```python
from build123d import *

# Parameters (mm, degrees)
SKETCH1_R           = 2
SKETCH1_R_2         = 2.5
SKETCH1_R_3         = 5.5
SKETCH1_R_4         = 1.75
SKETCH1_R_5         = 8.75
SKETCH1_R_6         = 16
BOSS_EXTRUDE1_DEPTH = 3


with BuildPart() as part:
    # Sketch1 → Boss-Extrude1 (new body)
    with BuildSketch(Plane.XY):
        with BuildLine():
            Line((-101.659864494, -83.45932429), (74.802197756, -41.852361745))
            ThreePointArc((74.802197756, -41.852361745), (107.704647438, 4.436019045), (66.002975735, 42.986712534))
            Line((66.002975735, 42.986712534), (-115.241855356, 47.493510774))
            ThreePointArc((-115.241855356, 47.493510774), (-132.576190146, 39.08356421), (-135.758964721, 20.081556162))
            ThreePointArc((-135.758964721, 20.081556162), (-135.373925263, 12.354995282), (-138.890242706, 5.464167316))
            ThreePointArc((-138.890242706, 5.464167316), (-145.2866753, -12.223575588), (-137.542861296, -29.364285714))
            ThreePointArc((-137.542861296, -29.364285714), (-135.311942722, -31.117537591), (-132.790777729, -32.419312113))
            ThreePointArc((-132.790777729, -32.419312113), (-124.308939641, -41.145198886), (-125.08868845, -53.289113787))
            ThreePointArc((-125.08868845, -53.289113787), (-123.065402539, -75.899910202), (-101.659864494, -83.45932429))
        make_face()
        with Locations((-128.3, -22.75)):
            Circle(SKETCH1_R, mode=Mode.SUBTRACT)
        with Locations((-68.3, -21.5)):
            Circle(SKETCH1_R_2, mode=Mode.SUBTRACT)
        with Locations((-128.3, -5.25)):
            Circle(SKETCH1_R, mode=Mode.SUBTRACT)
        with Locations((-74.1, 1.7)):
            Circle(SKETCH1_R_2, mode=Mode.SUBTRACT)
        with Locations((18.7, -8.7)):
            Circle(SKETCH1_R_2, mode=Mode.SUBTRACT)
        with Locations((76.2, -22)):
            Circle(SKETCH1_R_2, mode=Mode.SUBTRACT)
        with Locations((8.2, 8.3)):
            Circle(SKETCH1_R_2, mode=Mode.SUBTRACT)
        with Locations((64.934076539, 0)):
            Circle(SKETCH1_R_3, mode=Mode.SUBTRACT)
        with Locations((78.2, -0.1)):
            Circle(SKETCH1_R_2, mode=Mode.SUBTRACT)
        with Locations((-114.319590013, 12.574697906)):
            Circle(SKETCH1_R_4, mode=Mode.SUBTRACT)
        with Locations((-129.68917795, 25.055714157)):
            Circle(SKETCH1_R_4, mode=Mode.SUBTRACT)
        with Locations((-65.3, 20)):
            Circle(SKETCH1_R_2, mode=Mode.SUBTRACT)
        with Locations((-115.763875856, 26.5)):
            Circle(SKETCH1_R_5, mode=Mode.SUBTRACT)
        with Locations((-101.838573763, 27.944285843)):
            Circle(SKETCH1_R_4, mode=Mode.SUBTRACT)
        with Locations((-117.208161699, 40.425302094)):
            Circle(SKETCH1_R_4, mode=Mode.SUBTRACT)
        with Locations((28.1, 9)):
            Circle(SKETCH1_R_2, mode=Mode.SUBTRACT)
        with Locations((73.2, 22.3)):
            Circle(SKETCH1_R_2, mode=Mode.SUBTRACT)
        with Locations((-106.479181151, -63.019799174)):
            Circle(SKETCH1_R_6, mode=Mode.SUBTRACT)
    extrude(amount=BOSS_EXTRUDE1_DEPTH)


solid = part.part
```
Geometry: final body of the model. Coordinates: model frame, mm. Round coordinates to 2 decimals unless told otherwise and drop trailing zeros. Order: outer loops, then holes, each group sorted by start corner. A loop starts at its lowest first (then second) coordinate and runs counter-clockwise, first axis right, second up. Notation, with made-up numbers: (-1.5, 34.25) -> (52.5, 34.25) arc R16 cw to (52.5, 46.25) -> close; hole circle Ø11 at (5.25, 70). An arc over 180 degrees is marked (long way). Use one line per item in the form item = value.
(1) Section B-B on z = 0.85. Count the separate pieces of the cut face and the enclosed holes in it, and give its area (3 significant figures).
Results list:
separate_pieces = 1
enclosed_holes = 18
area = 23,800 mm^2
(2) Section A-A on y = -49.5. Return loops of the section in (x, z).
Results list:
outline = (-123.72, 0) -> (-115.04, 0) -> (-115.04, 3) -> (-123.72, 3) -> close; (-97.92, 0) -> (42.37, 0) -> (42.37, 3) -> (-97.92, 3) -> close
(3) First-contact query: pin 1 Ø1.5 at (x, z) = (-73, 1) entering from +Y. Flat tip, straight axial feed; report the tip coordinate or a pass-through.
Results list:
pin_1 = 46.46
(4) Section D-D on x = -55. Return loops of the section in (y, z).
Results list:
outline = (-72.46, 0) -> (46, 0) -> (46, 3) -> (-72.46, 3) -> close
(5) Section C-C on x = 89.5. Return loops of the section in (y, z), and give its area (3 significant figures).
Results list:
outline = (-35.29, 0) -> (35.29, 0) -> (35.29, 3) -> (-35.29, 3) -> close
area = 212 mm^2
(6) Ray query, probe 1 along X at (y, z) = (-1, 0.75); probe 2 along Y at (x, z) = (74.5, 0.8); probe 3 along Y at (x, z) = (-113, 2.4). Return the intervals inside material, ascending. Write a range as [from, to].
Results list:
probe_1 = [-143.1, 59.53], [70.34, 75.87], [80.53, 107.92]
probe_2 = [-41.92, -23.83], [-20.17, 20.16], [24.44, 41.92]
probe_3 = [-82.98, -77.63], [-48.41, 11.43], [13.72, 18.2], [34.8, 47.44]
(7) Draft query along X for faces 1 (the face through (107.786, 3.571, 1.479)), 2 (the face through (-20, -3, 3)), 3 (the face through (29.25, 6.78, 1.48)). Return one class per face: pulls with the +X half, pulls with the -X half, needs draft (parallel to the pull), parting line crosses it, or undercut.
Results list:
face_1 = pulls with the +X half
face_2 = needs draft
face_3 = undercut
